from build123d import *

# Parameters (mm, degrees)
F0_R     = 15
F0_R_2   = 13.75
F1_DEPTH = 6
F0_R_3   = 11
F2_DEPTH = 2
F3_DEPTH = 20
F4_R     = 1


with BuildPart() as f1:
    # F0 (on Top) → F1 (new body)
    with BuildSketch(Plane.XY):
        Circle(F0_R)
        Circle(F0_R_2, mode=Mode.SUBTRACT)
    extrude(amount=F1_DEPTH)

    # F0 (on Top) → F2 (join)
    with BuildSketch(Plane.XY):
        Circle(F0_R)
        Circle(F0_R_2, mode=Mode.SUBTRACT)
        Circle(F0_R_2)
        Circle(F0_R_3, mode=Mode.SUBTRACT)
        Circle(F0_R_3)
    extrude(amount=-F2_DEPTH)

    # F0 (on Top) → F3 (join)
    with BuildSketch(Plane.XY):
        Circle(F0_R_3)
    extrude(amount=F3_DEPTH)

    # F4
    f4_edges = [f1.edges().sort_by_distance(p)[0] for p in [
        (-11, 0, 20),
    ]]
    fillet(f4_edges, radius=F4_R)


solid = f1.part
The model under review builds one solid part; all positions refer to its coordinate system, in mm. A direction names the side the tool comes from. Give positions to 0.01 mm unless a question says otherwise; leave off trailing zeros. Write each loop counter-clockwise with the first axis right and the second up, starting at its lowest first coordinate (ties: lowest second). Pieces come first, ordered by that corner, then holes. Notation, with made-up numbers: M -20.5,46.25 L 18.5,46.25 A26 cw 18.5,74.25 Z; hole C 42.5,-39 d11. An arc over 180 degrees is marked long. One line per question, with ' | ' between items. Start each with the question number.
Item 1: We need section A-A on x = 0. Write out the cut boundary in (y, z), plus the area to 3 significant figures.
Item 2: Draft analysis for pull direction X (two halves, no side actions). For faces 1 (the flat face through (0, 0, -2)), 2 (the cylindrical face through (-2.981, -13.423, 2.958)), 3 (the cylindrical face through (-14.985, 0.66, 2.056)), 4 (the cylindrical face through (-2.38, -10.74, 9.37)), state which applies: released by +X, released by -X, zero draft, split by the parting line, or undercut.
Item 3: Wall thickness on line 1 (Y direction, x = 0, z = 2.65); line 2 (X direction, y = -4, z = 2.75); line 3 (Y direction, x = 10, z = 5.25): over which ranges is each line inside the solid? List them lowest first. Write a range as from..to.
Item 4: We need section D-D on z = 9.5. Write out the cut boundary in (x, y).
Item 5: For faces 5 (the flat face through (0, 0, 20)), 6 (the flat face through (-0.1, 11.3, 0)), list the 3-axis set-ups (+Z, -Z, +X, -X, +Y, -Y) from which the entire face can be reached by the end or side of a thin tool; tool diameter is ignored.
Item 6: We need section C-C on z = 1. Write out the cut boundary in (x, y).
Item 7: For pin 1 (6 mm diameter, centred on x = -4, z = 17.5, fed in from +Y); pin 2 (5 mm diameter, centred on y = -8, z = 16.5, fed in from +X); pin 3 (2 mm diameter, centred on x = 0, z = 12.5, fed in from -Y), all flat-tipped, find the tip position at first contact; note any pin that passes through.
Results found:
1) outline: M -15,-2 L 15,-2 L 15,6 L 13.75,6 L 13.75,0 L 11,0 L 11,19 A1 ccw 10,20 L -10,20 A1 ccw -11,19 L -11,0 L -13.75,0 L -13.75,6 L -15,6 Z | area: 515 mm2
2) face 1: zero draft | face 2: undercut | face 3: split by the parting line | face 4: undercut
3) line 1: y = -15..-13.75, -11..11, 13.75..15 | line 2: x = -14.46..-13.16, -10.25..10.25, 13.16..14.46 | line 3: y = -11.18..-9.44, -4.58..4.58, 9.44..11.18
4) outline: C 0,0 d22
5) face 5: +Z, +X, -X, +Y, -Y | face 6: +Z
6) outline: C 0,0 d30; C 0,0 d22; hole C 0,0 d27.5
7) pin 1: stops at y = 10.95 | pin 2: stops at x = 9.53 | pin 3: stops at y = -11
